Input: part model. Units: mm. Frame: model coordinates. Face numbers are marked on the shaded views. A direction names the side the tool comes from. Coordinates: 2 decimals unless noted, no trailing zeros. Loops run counter-clockwise (first coordinate to the right, second up) from the corner with the lowest first, then second, coordinate; pieces in that order, holes last.
(1) Contact query for flat-ended pins moving along their axis: P1, Ø4, axis at y = 37, z = -2, coming from the +X side; P2, Ø10, axis at x = -10, y = 20.5, coming from the -Z side; P3, Ø16, axis at x = 0, z = 0, coming from the -Y side. Output: stop coordinate, or through.
(2) Section A-A, the plane z = 0. Return loops of the section in (x, y).
(3) Section C-C, the plane y = 18. Return loops of the section in (x, z), then the cut area to 3 significant figures.
(4) Mould query, pull axis X, two halves, no side actions, for the marked faces 3, 4, 5 and 6. Classes: released by +X, released by -X, zero draft, split by the parting line, or undercut.
(5) Section B-B, the plane x = 0. Return loops of the section in (y, z).
(6) Section D-D, the plane z = 9.5. Return loops of the section in (x, y).
(7) Set-up query: the marked faces 1 and 2. Return all of +Z, -Z, +X, -X, +Y, -Y with unobstructed straight access to the full face (end or side cutting, diameter ignored); none if empty.
(8) Line query: L1, parallel to X at y = 43, z = 0; L2, parallel to X at y = 13, z = 0; L3, parallel to Z at x = -1, y = 4.5. Output: solid intervals per line, ascending.
```python
from build123d import *

# Parameters (mm, degrees)
SKETCH1_R           = 22
SKETCH1_R_2         = 5
BOSS_EXTRUDE1_DEPTH = 44
SKETCH2_R           = 15
CUT_EXTRUDE1_DEPTH  = 4
CUT_EXTRUDE2_START  = -4
SKETCH3_R           = 15
CUT_EXTRUDE2_DEPTH  = 4


with BuildPart() as part:
    # Sketch1 → Boss-Extrude1 (new body)
    with BuildSketch(Plane(origin=(0, 0, 0), x_dir=(1, 0, 0), z_dir=(0, 1, 0))):
        with Locations(Location((0, 0, 0), (0, 0, 270))):
            Circle(SKETCH1_R)
        with Locations(Location((0, 0, 0), (0, 0, 270))):
            Circle(SKETCH1_R_2, mode=Mode.SUBTRACT)
    extrude(amount=BOSS_EXTRUDE1_DEPTH)

    # Sketch2 → Cut-Extrude1 (cut)
    with BuildSketch(Plane(origin=(0, 44, 0), x_dir=(1, 0, 0), z_dir=(0, 1, 0))):
        with Locations(Location((0, 0, 0), (0, 0, 270))):
            Circle(SKETCH2_R)
    extrude(amount=-CUT_EXTRUDE1_DEPTH, mode=Mode.SUBTRACT)

    # Sketch3 → Cut-Extrude2 (cut)
    with BuildSketch(Plane.XZ.offset(CUT_EXTRUDE2_START)):
        with Locations(Location((0, 0, 0), (0, 0, 90))):
            Circle(SKETCH3_R)
    extrude(amount=CUT_EXTRUDE2_DEPTH, mode=Mode.SUBTRACT)


solid = part.part
```
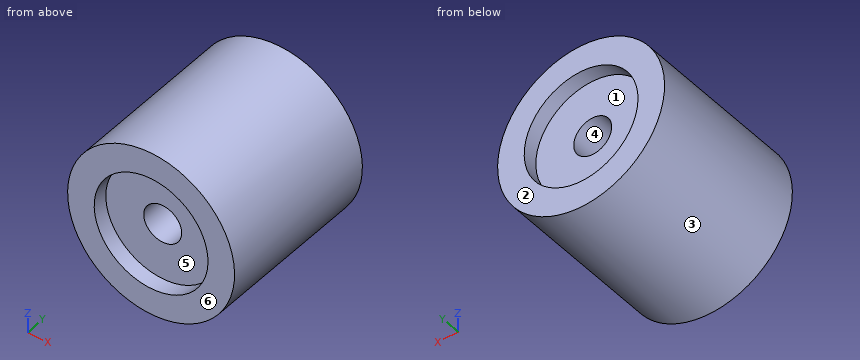
Report:
1. P1: stops at x = 22
1. P2: stops at z = -21.42
1. P3: stops at y = 4
2. outline: (-22, 0) - (-15, 0) - (-15, 4) - (-5, 4) - (-5, 40) - (-15, 40) - (-15, 44) - (-22, 44) - close; (5, 4) - (15, 4) - (15, 0) - (22, 0) - (22, 44) - (15, 44) - (15, 40) - (5, 40) - close
3. outline: circle Ø44 at (0, 0); hole circle Ø10 at (0, 0)
3. area: 1,440 mm2
4. face 3: split by the parting line
4. face 4: undercut
4. face 5: undercut
4. face 6: zero draft
5. outline: (0, -22) - (44, -22) - (44, -15) - (40, -15) - (40, -5) - (4, -5) - (4, -15) - (0, -15) - close; (0, 15) - (4, 15) - (4, 5) - (40, 5) - (40, 15) - (44, 15) - (44, 22) - (0, 22) - close
6. outline: (-19.84, 0) - (-11.61, 0) - (-11.61, 4) - (11.61, 4) - (11.61, 0) - (19.84, 0) - (19.84, 44) - (11.61, 44) - (11.61, 40) - (-11.61, 40) - (-11.61, 44) - (-19.84, 44) - close
7. face 1: +Y
7. face 2: +Z, -Z, +X, -X, +Y
8. L1: x = -22 to -15, 15 to 22
8. L2: x = -22 to -5, 5 to 22
8. L3: z = -21.98 to -4.9, 4.9 to 21.98
